Read the model definition and answer for the solid it produces. Units are mm, in the model's axes. Face numbers are marked on the shaded views. A direction names the side the tool comes from. Coordinates: 2 decimals unless noted, no trailing zeros. Write each loop counter-clockwise with the first axis right and the second up, starting at its lowest first coordinate (ties: lowest second). Pieces come first, ordered by that corner, then holes. Notation, with made-up numbers: M 66.5,-24.75 L 72.5,-24.75 A20 ccw 72.5,-15.75 Z; hole C 21.25,86 d4. An arc over 180 degrees is marked long. Use a Markdown table: item, result. Add a question column.
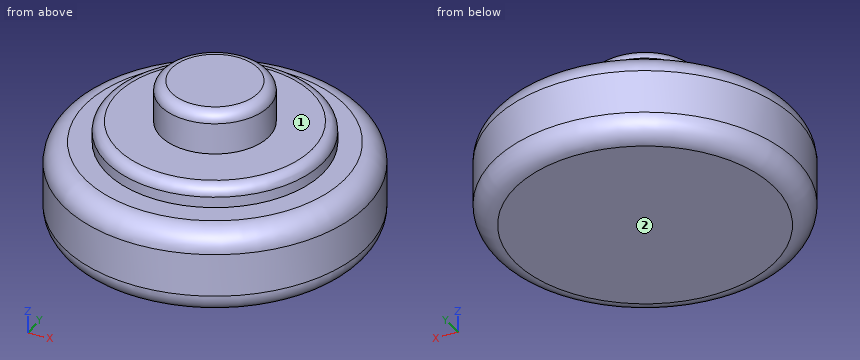
from build123d import *

# Parameters (mm, degrees)
CYLINDER001_R     = 11.1125
CYLINDER001_DEPTH = 6.35
FILLET006_R       = 1.5875
FILLET007_R       = 1.5875
SKETCH003_R       = 7.9375
PAD003_DEPTH      = 1.5875
FILLET008_R       = 0.79375
SKETCH004_R       = 3.96875
PAD004_DEPTH      = 3.1
FILLET009_R       = 0.79375


with BuildPart() as part:
    # Cylinder001 → Cylinder001 (new body)
    with BuildSketch(Plane.XY):
        Circle(CYLINDER001_R)
    extrude(amount=CYLINDER001_DEPTH)

    # Fillet006
    fillet006_edges = [part.edges().sort_by_distance(p)[0] for p in [
        (-11.1125, 0, 6.35),
    ]]
    fillet(fillet006_edges, radius=FILLET006_R)

    # Fillet007
    fillet007_edges = [part.edges().sort_by_distance(p)[0] for p in [
        (-11.1125, 0, 0),
    ]]
    fillet(fillet007_edges, radius=FILLET007_R)

    # Sketch003 → Pad003 (new body)
    with BuildSketch(Plane.XY.offset(6.35)):
        Circle(SKETCH003_R)
    extrude(amount=PAD003_DEPTH)

    # Fillet008
    fillet008_edges = [part.edges().sort_by_distance(p)[0] for p in [
        (-7.9375, 0, 7.9375),
    ]]
    fillet(fillet008_edges, radius=FILLET008_R)

    # Sketch004 → Pad004 (new body)
    with BuildSketch(Plane.XY.offset(7.9375)):
        Circle(SKETCH004_R)
    extrude(amount=PAD004_DEPTH)

    # Fillet009
    fillet009_edges = [part.edges().sort_by_distance(p)[0] for p in [
        (-3.96875, 0, 11.0375),
    ]]
    fillet(fillet009_edges, radius=FILLET009_R)


solid = part.part
Item 1: Each of these flat-tipped pins is pushed along its axis until it touches: pin 1 (5 mm diameter, centred on x = 1.5, z = 9, fed in from +Y); pin 2 (2 mm diameter, centred on x = 1, z = 10, fed in from +Y); pin 3 (1 mm diameter, centred on x = -6, z = 8, fed in from +Y). Where does it stop, or does it pass through?
Item 2: For the marked faces 1 and 2, determine the directions among +Z, -Z, +X, -X, +Y, -Y from which every point of the face is accessible in a straight line to the end or side of a thin tool.
Item 3: Find section D-D on z = 8.5. Give the vertices of the cut face in (x, y).
Item 4: Find section C-C on z = 3.25. Give the vertices of the cut face in (x, y) (1 decimal).
Item 5: Consider probe 1 along Z at (x, y) = (-4.75, 2); probe 2 along Z at (x, y) = (2, -8.75); probe 3 along X at (y, z) = (3.25, 9). Determine where each line is inside the solid, lowest interval first.
Geometry says:
| question | item | result |
|---|---|---|
| 1 | pin 1 | stops at y = 7.94 |
| 1 | pin 2 | stops at y = 3.97 |
| 1 | pin 3 | stops at y = 5.32 |
| 2 | face 1 | +Z |
| 2 | face 2 | -Z, +X, -X, +Y, -Y |
| 3 | outline | C 0,0 d7.94 |
| 4 | outline | C 0,0 d22.2 |
| 5 | probe 1 | z = 0 to 7.94 |
| 5 | probe 2 | z = 0 to 6.35 |
| 5 | probe 3 | x = -2.28 to 2.28 |
